Source: CAD feature listing. Evaluate the final solid. Frame: model axes, mm. A direction names the side the tool comes from. Round coordinates to 2 decimals unless told otherwise and drop trailing zeros. Loops run counter-clockwise (first coordinate to the right, second up) from the corner with the lowest first, then second, coordinate; pieces in that order, holes last. Notation, with made-up numbers: (26.25, 81) -> (66.25, 81) arc R15 cw to (66.25, 89) -> close; hole circle Ø3 at (-33.75, 17.5). An arc over 180 degrees is marked (long way). Put each result on its own line as item: value. Start each with the question number.
1. Material intervals for L1, parallel to X at y = 27.5, z = 52.5 (3 decimals); L2, parallel to Y at x = -18, z = 1.8 (3 decimals); L3, parallel to X at y = -25, z = 11, sorted ascending.
2. Cut plane B-B (x = -18). Return the cut outline in (y, z) (3 decimals).
3. Set-up query: faces 4 (the flat face through (-41.365, 25, 55)), 5 (the cylindrical face through (21.114, 20.981, 2.465)), 6 (the flat face through (17, 21, 35)), 7 (the flat face through (0, -29, 35)). Return all of +Z, -Z, +X, -X, +Y, -Y with unobstructed straight access to the full face (end or side cutting, diameter ignored); none if empty.
4. Cut plane A-A (y = -22). Return the cut outline in (x, z) (3 decimals).
5. Cut plane C-C (x = -38.1). Return the cut outline in (y, z) (3 decimals).
6. Draft query along Y for faces 1 (the flat face through (17, 12.5, 20)), 2 (the cylindrical face through (-14.886, 20.981, 2.465)), 3 (the flat face through (8.5, 21, 20)). Return one class per face: pulls with the +Y half, pulls with the -Y half, needs draft (parallel to the pull), parting line crosses it, or undercut.
7. Contact query for flat-ended pins moving along their axis: pin 1 (12 mm diameter, centred on y = -23, z = 37.5, fed in from +X); pin 2 (12 mm diameter, centred on x = 12.5, z = 9.5, fed in from +Y); pin 3 (10 mm diameter, centred on y = -33, z = 32.5, fed in from -X); pin 4 (8.5 mm diameter, centred on x = 0, y = -28, fed in from -Z). Output: stop coordinate, or through.
8. Cut plane D-D (y = -1.5). Return the cut outline in (x, z) (3 decimals).
```python
from build123d import *

# Parameters (mm, degrees)
F0_W      = 52
F0_H      = 67.66
F2_DEPTH  = 5
F1_R      = 3.265
F3_DEPTH  = 5
F4_W      = 52
F4_H      = 67.66
F5_DEPTH  = 30
F6_W      = 17.5
F6_H      = 17.5
F6_W_2    = 25
F7_DEPTH  = 30
F8_W      = 52
F8_H      = 67.66
F9_DEPTH  = 25
F10_W     = 100
F10_H     = 100
F11_DEPTH = 10
F13_DEPTH = 10


with BuildPart() as f2:
    # F0 (on Top) → F2 (new body)
    with BuildSketch(Plane.XY):
        with Locations((0, -3.83)):
            Rectangle(F0_W, F0_H)
    extrude(amount=F2_DEPTH)

    # F1 (on face) → F3 (cut)
    with BuildSketch(Plane.XY):
        with Locations((-18, 20)):
            Circle(F1_R)
        with Locations((18, 20)):
            Circle(F1_R)
        with Locations((0, -28)):
            Circle(F1_R)
    extrude(amount=F3_DEPTH, mode=Mode.SUBTRACT)

    # F4 (on face) → F5 (join)
    with BuildSketch(Plane.XY.offset(5)):
        with Locations((0, -3.83)):
            Rectangle(F4_W, F4_H)
    extrude(amount=F5_DEPTH)

    # F6 (on face) → F7 (cut)
    with BuildSketch(Plane.XY.offset(35)):
        with Locations((-17.25, 21.25)):
            Rectangle(F6_W, F6_H)
        with Locations((17.25, 21.25)):
            Rectangle(F6_W, F6_H)
        with Locations((0, -28.91)):
            Rectangle(F6_W_2, F6_H)
    extrude(amount=-F7_DEPTH, mode=Mode.SUBTRACT)

    # F8 (on face) → F9 (join)
    with BuildSketch(Plane.XY.offset(35)):
        with Locations((0, -3.83)):
            Rectangle(F8_W, F8_H)
    extrude(amount=F9_DEPTH)

    # F10 (on face) → F11 (join)
    with BuildSketch(Plane.XY.offset(60)):
        Rectangle(F10_W, F10_H)
    extrude(amount=-F11_DEPTH)

    # F12 (on face) → F13 (cut)
    with BuildSketch(Plane.XY.offset(60)):
        with BuildLine():
            Line((34.835, -6.35), (41.365, -6.35))
            ThreePointArc((41.365, -6.35), (38.1, -3.085), (34.835, -6.35))
        make_face()
        with BuildLine():
            ThreePointArc((34.835, -6.35), (38.1, -9.615), (41.365, -6.35))
            Line((41.365, -6.35), (34.835, -6.35))
        make_face()
        with BuildLine():
            ThreePointArc((34.835, -6.35), (38.1, -3.085), (41.365, -6.35))
            Line((41.365, -6.35), (41.365, 6.35))
            ThreePointArc((41.365, 6.35), (38.1, 3.085), (34.835, 6.35))
            Line((34.835, 6.35), (34.835, -6.35))
        make_face()
        with BuildLine():
            Line((34.835, 6.35), (41.365, 6.35))
            ThreePointArc((41.365, 6.35), (38.1, 9.615), (34.835, 6.35))
        make_face()
        with BuildLine():
            ThreePointArc((34.835, 6.35), (38.1, 3.085), (41.365, 6.35))
            Line((41.365, 6.35), (34.835, 6.35))
        make_face()
        with BuildLine():
            Line((34.835, -31.75), (41.365, -31.75))
            ThreePointArc((41.365, -31.75), (38.1, -28.485), (34.835, -31.75))
        make_face()
        with BuildLine():
            ThreePointArc((34.835, -31.75), (38.1, -35.015), (41.365, -31.75))
            Line((41.365, -31.75), (34.835, -31.75))
        make_face()
        with BuildLine():
            ThreePointArc((34.835, -31.75), (38.1, -28.485), (41.365, -31.75))
            Line((41.365, -31.75), (41.365, -19.05))
            ThreePointArc((41.365, -19.05), (38.1, -22.315), (34.835, -19.05))
            Line((34.835, -19.05), (34.835, -31.75))
        make_face()
        with BuildLine():
            Line((34.835, -19.05), (41.365, -19.05))
            ThreePointArc((41.365, -19.05), (38.1, -15.785), (34.835, -19.05))
        make_face()
        with BuildLine():
            ThreePointArc((34.835, -19.05), (38.1, -22.315), (41.365, -19.05))
            Line((41.365, -19.05), (34.835, -19.05))
        make_face()
        with BuildLine():
            ThreePointArc((34.835, 31.75), (38.1, 28.485), (41.365, 31.75))
            ThreePointArc((41.365, 31.75), (38.1, 35.015), (34.835, 31.75))
        make_face()
        with BuildLine():
            Line((41.365, 19.05), (41.365, 31.75))
            ThreePointArc((41.365, 31.75), (38.1, 28.485), (34.835, 31.75))
            Line((34.835, 31.75), (34.835, 19.05))
            ThreePointArc((34.835, 19.05), (38.1, 22.315), (41.365, 19.05))
        make_face()
        with BuildLine():
            ThreePointArc((34.835, 19.05), (38.1, 15.785), (41.365, 19.05))
            ThreePointArc((41.365, 19.05), (38.1, 22.315), (34.835, 19.05))
        make_face()
        with BuildLine():
            ThreePointArc((-41.365, -31.75), (-38.1, -35.015), (-34.835, -31.75))
            ThreePointArc((-34.835, -31.75), (-38.1, -28.485), (-41.365, -31.75))
        make_face()
        with BuildLine():
            ThreePointArc((-41.365, -31.75), (-38.1, -28.485), (-34.835, -31.75))
            Line((-34.835, -31.75), (-34.835, -19.05))
            ThreePointArc((-34.835, -19.05), (-38.1, -22.315), (-41.365, -19.05))
            Line((-41.365, -19.05), (-41.365, -31.75))
        make_face()
        with BuildLine():
            ThreePointArc((-41.365, -19.05), (-38.1, -22.315), (-34.835, -19.05))
            ThreePointArc((-34.835, -19.05), (-38.1, -15.785), (-41.365, -19.05))
        make_face()
        with BuildLine():
            ThreePointArc((-41.365, -6.35), (-38.1, -9.615), (-34.835, -6.35))
            ThreePointArc((-34.835, -6.35), (-38.1, -3.085), (-41.365, -6.35))
        make_face()
        with BuildLine():
            ThreePointArc((-41.365, -6.35), (-38.1, -3.085), (-34.835, -6.35))
            Line((-34.835, -6.35), (-34.835, 6.35))
            ThreePointArc((-34.835, 6.35), (-38.1, 3.085), (-41.365, 6.35))
            Line((-41.365, 6.35), (-41.365, -6.35))
        make_face()
        with BuildLine():
            ThreePointArc((-41.365, 6.35), (-38.1, 3.085), (-34.835, 6.35))
            ThreePointArc((-34.835, 6.35), (-38.1, 9.615), (-41.365, 6.35))
        make_face()
        with BuildLine():
            ThreePointArc((-41.365, 19.05), (-38.1, 15.785), (-34.835, 19.05))
            ThreePointArc((-34.835, 19.05), (-38.1, 22.315), (-41.365, 19.05))
        make_face()
        with BuildLine():
            ThreePointArc((-41.365, 19.05), (-38.1, 22.315), (-34.835, 19.05))
            Line((-34.835, 19.05), (-34.835, 31.75))
            ThreePointArc((-34.835, 31.75), (-38.1, 28.485), (-41.365, 31.75))
            Line((-41.365, 31.75), (-41.365, 19.05))
        make_face()
        with BuildLine():
            ThreePointArc((-41.365, 31.75), (-38.1, 28.485), (-34.835, 31.75))
            ThreePointArc((-34.835, 31.75), (-38.1, 35.015), (-41.365, 31.75))
        make_face()
    extrude(amount=-F13_DEPTH, mode=Mode.SUBTRACT)


solid = f2.part
```
Solution:
1. L1: x = -50 to -41.365, -34.835 to 34.835, 41.365 to 50
1. L2: y = -37.66 to 16.735, 23.265 to 30
1. L3: x = -26 to -12.5, 12.5 to 26
2. outline: (-50, 50) -> (-37.66, 50) -> (-37.66, 0) -> (16.735, 0) -> (16.735, 5) -> (12.5, 5) -> (12.5, 35) -> (30, 35) -> (30, 50) -> (50, 50) -> (50, 60) -> (-50, 60) -> close; (23.265, 0) -> (30, 0) -> (30, 5) -> (23.265, 5) -> close
3. face 4: +Z, -Z
3. face 5: -Z
3. face 6: +X, +Y
3. face 7: -Y
4. outline: (-50, 50) -> (-41.365, 50) -> (-41.365, 60) -> (-50, 60) -> close; (-34.835, 50) -> (-26, 50) -> (-26, 0) -> (26, 0) -> (26, 50) -> (34.835, 50) -> (34.835, 60) -> (-34.835, 60) -> close; (41.365, 50) -> (50, 50) -> (50, 60) -> (41.365, 60) -> close; hole (-12.5, 5) -> (12.5, 5) -> (12.5, 35) -> (-12.5, 35) -> close
5. outline: (-50, 50) -> (-35.015, 50) -> (-35.015, 60) -> (-50, 60) -> close; (-15.785, 50) -> (-9.615, 50) -> (-9.615, 60) -> (-15.785, 60) -> close; (9.615, 50) -> (15.785, 50) -> (15.785, 60) -> (9.615, 60) -> close; (35.015, 50) -> (50, 50) -> (50, 60) -> (35.015, 60) -> close
6. face 1: pulls with the +Y half
6. face 2: undercut
6. face 3: needs draft
7. pin 1: stops at x = 26
7. pin 2: stops at y = 30
7. pin 3: stops at x = -26
7. pin 4: stops at z = 0
8. outline: (-50, 50) -> (-41.365, 50) -> (-41.365, 60) -> (-50, 60) -> close; (-34.835, 50) -> (-26, 50) -> (-26, 0) -> (26, 0) -> (26, 50) -> (34.835, 50) -> (34.835, 60) -> (-34.835, 60) -> close; (41.365, 50) -> (50, 50) -> (50, 60) -> (41.365, 60) -> close
